```python
from build123d import *

# Parameters (mm, degrees)
F0_R     = 17.49425
F1_DEPTH = 5.1308
F2_R     = 5.55625
F3_DEPTH = 152
F4_R     = 4.318
F5_DEPTH = 157.1318
F7_D     = 5.1308


with BuildPart() as f1:
    # F0 (on Top) → F1 (new body)
    with BuildSketch(Plane.XY):
        Circle(F0_R)
    extrude(amount=F1_DEPTH)

    # F2 (on face) → F3 (join)
    with BuildSketch(Plane.XY.offset(5.1308)):
        Circle(F2_R)
    extrude(amount=F3_DEPTH)

    # F4 (on face) → F5 (cut, through all)
    with BuildSketch(Plane(origin=(0, 0, 0), x_dir=(1, 0, 0), z_dir=(0, 0, -1))):
        Circle(F4_R)
    extrude(amount=-F5_DEPTH, mode=Mode.SUBTRACT)

    # F7 (through all)
    with Locations(Plane(origin=(0, 0, 0), x_dir=(1, 0, 0), z_dir=(0, 0, -1))):
        with Locations((-12.7, 0), (12.7, 0)):
            Hole(F7_D / 2)


solid = f1.part
```
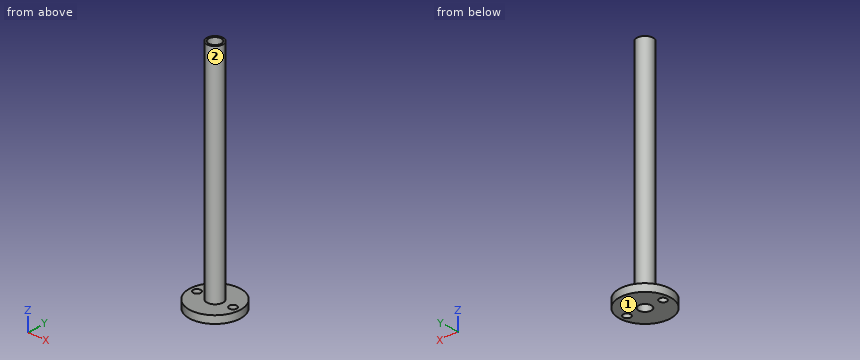
Input: part model. Units: mm. Frame: model coordinates. Face numbers are marked on the shaded views. A direction names the side the tool comes from. Round coordinates to 2 decimals unless told otherwise and drop trailing zeros. Loops run counter-clockwise (first coordinate to the right, second up) from the corner with the lowest first, then second, coordinate; pieces in that order, holes last. Notation, with made-up numbers: (15, 75.5) -> (52, 75.5) arc R19 ccw to (52, 87.5) -> close; hole circle Ø2 at (70, 0). An arc over 180 degrees is marked (long way). Write each question's results on one line, items separated by ' | '.
1. Set-up query: the marked faces 1 and 2. Return all of +Z, -Z, +X, -X, +Y, -Y with unobstructed straight access to the full face (end or side cutting, diameter ignored); none if empty.
Geometry results:
face 1: -Z, +X, -X, +Y, -Y | face 2: +Z
2. Section D-D (x = 12.7). Return loops of the section in (y, z), and give its area (3 significant figures).
Geometry results:
outline: (-12.03, 0) -> (-2.57, 0) -> (-2.57, 5.13) -> (-12.03, 5.13) -> close; (2.57, 0) -> (12.03, 0) -> (12.03, 5.13) -> (2.57, 5.13) -> close | area: 97.1 mm2
3. Section B-B (y = 0). Return loops of the section in (x, z).
Geometry results:
outline: (-17.49, 0) -> (-15.27, 0) -> (-15.27, 5.13) -> (-17.49, 5.13) -> close; (-10.13, 0) -> (-4.32, 0) -> (-4.32, 157.13) -> (-5.56, 157.13) -> (-5.56, 5.13) -> (-10.13, 5.13) -> close; (4.32, 0) -> (10.13, 0) -> (10.13, 5.13) -> (5.56, 5.13) -> (5.56, 157.13) -> (4.32, 157.13) -> close; (15.27, 0) -> (17.49, 0) -> (17.49, 5.13) -> (15.27, 5.13) -> close
4. Section C-C (z = 45). Return loops of the section in (x, y), and give its area (3 significant figures).
Geometry results:
outline: circle Ø11.11 at (0, 0); hole circle Ø8.64 at (0, 0) | area: 38.4 mm2
5. Ray query, line 1 (Y direction, x = -0.5, z = 51); line 2 (Y direction, x = 0, z = 69.5); line 3 (Z direction, x = 7.5, y = -1.5). Return the intervals inside material, ascending. Write a range as from..to.
Geometry results:
line 1: -5.53..-4.29, 4.29..5.53 | line 2: -5.56..-4.32, 4.32..5.56 | line 3: 0..5.13
6. First-contact query: P1, Ø6, axis at x = -13.5, y = 11, coming from the +Z side; P2, Ø12, axis at y = 0.5, z = 65.5, coming from the -X side; P3, Ø3, axis at y = 4.5, z = 112, coming from the -X side. Flat tips, straight axial feed; report the tip coordinate or a pass-through.
Geometry results:
P1: z = 5.13 | P2: x = -5.56 | P3: x = -4.68
7. Section A-A (x = 0). Return loops of the section in (y, z).
Geometry results:
outline: (-17.49, 0) -> (-4.32, 0) -> (-4.32, 157.13) -> (-5.56, 157.13) -> (-5.56, 5.13) -> (-17.49, 5.13) -> close; (4.32, 0) -> (17.49, 0) -> (17.49, 5.13) -> (5.56, 5.13) -> (5.56, 157.13) -> (4.32, 157.13) -> close
